The model under review builds one solid part; all positions refer to its coordinate system, in mm. Face numbers are marked on the shaded views. A direction names the side the tool comes from. Coordinates: 2 decimals unless noted, no trailing zeros. Order: outer loops, then holes, each group sorted by start corner. A loop starts at its lowest first (then second) coordinate and runs counter-clockwise, first axis right, second up. Notation, with made-up numbers: M -5,58.5 L 4,58.5 A16 ccw 4,81.5 Z; hole C 79.5,43.5 d1. An arc over 180 degrees is marked long. One line per item, written item: value.
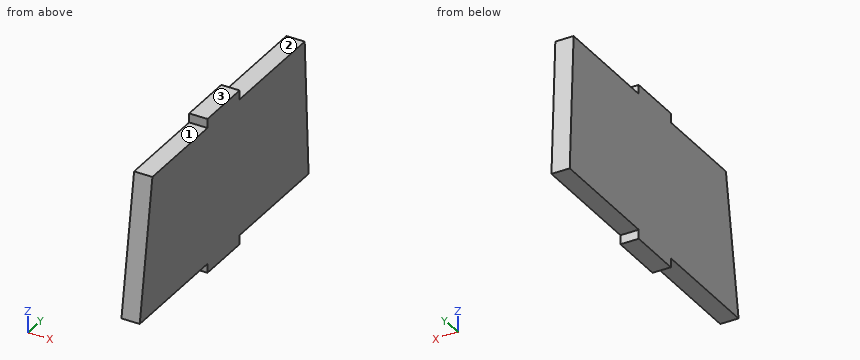
```python
from build123d import *

# Parameters (mm, degrees)
SKETCH1_W           = 12.7
SKETCH1_H           = 76.2
SKETCH1_W_2         = 190.5
BOSS_EXTRUDE1_DEPTH = 25.4


with BuildPart() as part:
    # Sketch1 → Boss-Extrude1 (new body)
    with BuildSketch(Plane(origin=(0, 0, 0), x_dir=(0, 0, -1), z_dir=(1, 0, 0))):
        Polygon((95.25, 201.879837032), (-95.25, 192.69579571), (-95.25, 38.1), (95.25, 38.1), align=None)
        with Locations((101.6, 0)):
            Rectangle(SKETCH1_W, SKETCH1_H)
        Rectangle(SKETCH1_W_2, SKETCH1_H)
        with Locations((-101.6, 0)):
            Rectangle(SKETCH1_W, SKETCH1_H)
        Polygon((95.25, -38.1), (-95.25, -38.1), (-95.25, -168.80022374), (95.25, -198.895286486), align=None)
    extrude(amount=BOSS_EXTRUDE1_DEPTH)


solid = part.part
```
(1) Tool access review of the marked faces 1, 2 and 3: name each direction out of +Z, -Z, +X, -X, +Y, -Y from which nothing blocks a thin tool from reaching the whole face with its end or side.
Geometry results:
face 1: +Z, +X, -X, -Y
face 2: +Z, +X, -X, +Y
face 3: +Z, +X, -X, +Y, -Y
(2) We need section B-B, the plane y = 107. State the section outline as (x, z) points, plus the area to 3 significant figures.
Geometry results:
outline: M 0,-95.25 L 25.4,-95.25 L 25.4,95.25 L 0,95.25 Z
area: 4,840 mm2
(3) Insertion check: pin 1 Ø10 at (x, z) = (12.5, 103.5) entering from +Y; pin 2 Ø10 at (x, z) = (12.5, 26) entering from -Y; pin 3 Ø5 at (x, z) = (3, 29.5) entering from -Y. Each pin has a flat end and moves straight along its axis. Give the tip position at first contact, or say it passes through.
Geometry results:
pin 1: stops at y = 38.1
pin 2: stops at y = -180.53
pin 3: stops at y = -179.58
(4) For L1, parallel to Z at x = 23.5, y = 171; L2, parallel to Y at x = 3.5, z = -96; L3, parallel to Y at x = 7, z = 92, list the stretches that pass through material, from the lowest coordinate up.
Geometry results:
L1: z = -95.25 to 95.25
L2: y = -38.1 to 38.1
L3: y = -169.31 to 192.85
(5) We need section C-C, the plane z = 62.5. State the section outline as (x, y) points.
Geometry results:
outline: M 0,-173.97 L 25.4,-173.97 L 25.4,194.27 L 0,194.27 Z
(6) We need section A-A, the plane x = 16.25. State the section outline as (y, z) points.
Geometry results:
outline: M -198.9,-95.25 L -38.1,-95.25 L -38.1,-107.95 L 38.1,-107.95 L 38.1,-95.25 L 201.88,-95.25 L 192.7,95.25 L 38.1,95.25 L 38.1,107.95 L -38.1,107.95 L -38.1,95.25 L -168.8,95.25 Z
